Source: three-view drawing plus pictorial views. Frame: mm from the lowest corner of the part. A direction names the side the tool comes from. Round coordinates to 2 decimals unless told otherwise and drop trailing zeros. Loops run counter-clockwise (first coordinate to the right, second up) from the corner with the lowest first, then second, coordinate; pieces in that order, holes last. Notation, with made-up numbers: M 69,-31.75 L 95,-31.75 A14 ccw 95,-13.75 Z; hole C 65.5,5 d6. An arc over 180 degrees is marked long. Answer as a JSON object with one key per item and string values.
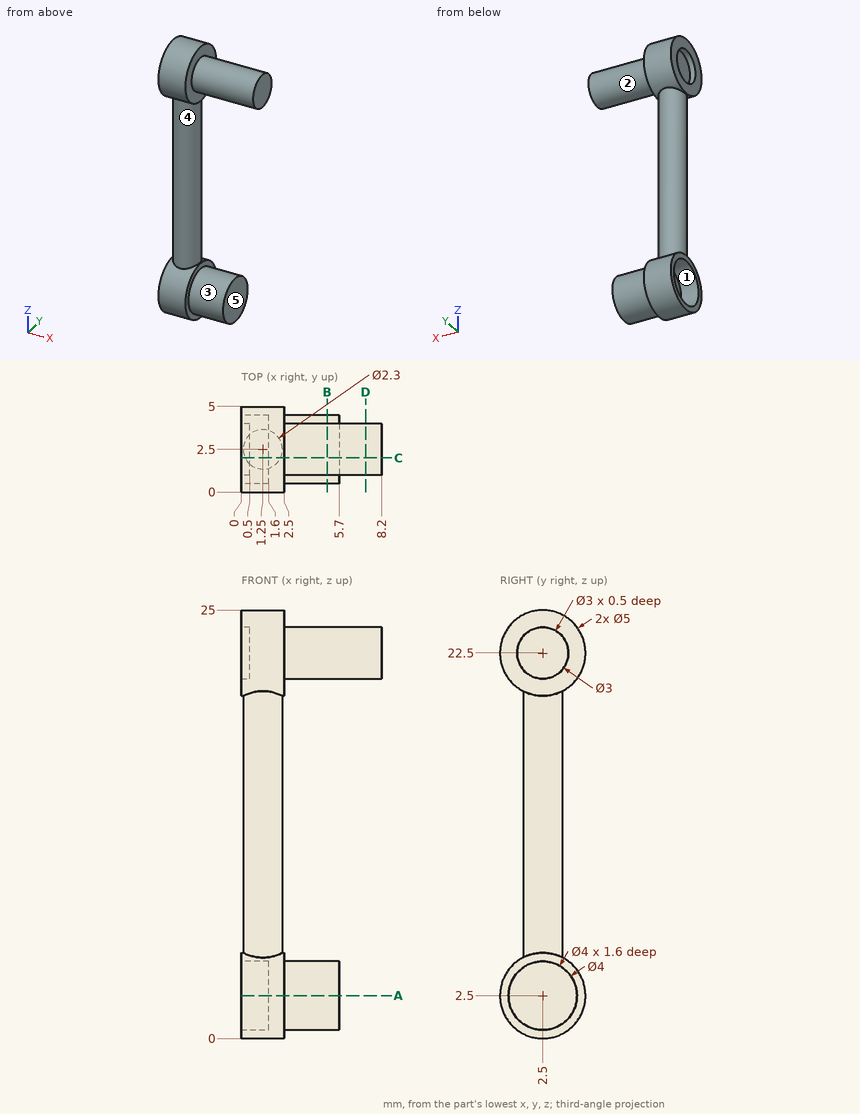
1) Line query: probe 1 along Y at (x, z) = (1.25, 5); probe 2 along Z at (x, y) = (4.25, 1.75); probe 3 along Z at (x, y) = (4.5, 2.25). Output: solid intervals per line, ascending.
Geometry results:
{"probe 1": "1.35 to 3.65", "probe 2": "0.65 to 4.35, 21.2 to 23.8", "probe 3": "0.52 to 4.48, 21.02 to 23.98"}
2) First-contact query: pin 1 (2.5 mm diameter, centred on y = 3.5, z = 1.5, fed in from +X); pin 2 (1.5 mm diameter, centred on y = 2.5, z = 22.5, fed in from -X); pin 3 (2 mm diameter, centred on x = 3, z = 10.5, fed in from -Y). Flat tips, straight axial feed; report the tip coordinate or a pass-through.
Geometry results:
{"pin 1": "x = 5.7", "pin 2": "x = 0.5", "pin 3": "y = 1.63"}
3) Set-up query: the marked faces 1 and 2. Return all of +Z, -Z, +X, -X, +Y, -Y with unobstructed straight access to the full face (end or side cutting, diameter ignored); none if empty.
Geometry results:
{"face 1": "-X", "face 2": "+X"}
4) Pull-direction query (Z, two-part tool) for the marked faces 3, 4 and 5; classes: +Z half, -Z half, draft (parallel to the pull), parting line (faces both ways), or undercut.
Geometry results:
{"face 3": "undercut", "face 4": "undercut", "face 5": "draft"}
5) Cut plane C-C on y = 2. Return the cut outline in (x, z), and give its area (3 significant figures).
Geometry results:
{"outline": "M 0,0.05 L 2.5,0.05 L 2.5,0.56 L 5.7,0.56 L 5.7,4.44 L 2.5,4.44 L 2.5,4.95 L 2.29,4.95 L 2.29,20.05 L 2.5,20.05 L 2.5,21.09 L 8.2,21.09 L 8.2,23.91 L 2.5,23.91 L 2.5,24.95 L 0,24.95 L 0,23.91 L 0.5,23.91 L 0.5,21.09 L 0,21.09 L 0,20.05 L 0.21,20.05 L 0.21,4.95 L 0,4.95 L 0,4.44 L 1.6,4.44 L 1.6,0.56 L 0,0.56 Z", "area": "76.7 mm2"}
6) Cut plane D-D on x = 7.25. Return the cut outline in (y, z).
Geometry results:
{"outline": "C 2.5,22.5 d3"}
7) Cut plane A-A on z = 2.5. Return the cut outline in (x, y).
Geometry results:
{"outline": "M 0,0 L 2.5,0 L 2.5,0.5 L 5.7,0.5 L 5.7,4.5 L 2.5,4.5 L 2.5,5 L 0,5 L 0,4.5 L 1.6,4.5 L 1.6,0.5 L 0,0.5 Z"}
8) Cut plane B-B on x = 5. Return the cut outline in (y, z), and give its area (3 significant figures).
Geometry results:
{"outline": "C 2.5,2.5 d4; C 2.5,22.5 d3", "area": "19.6 mm2"}
